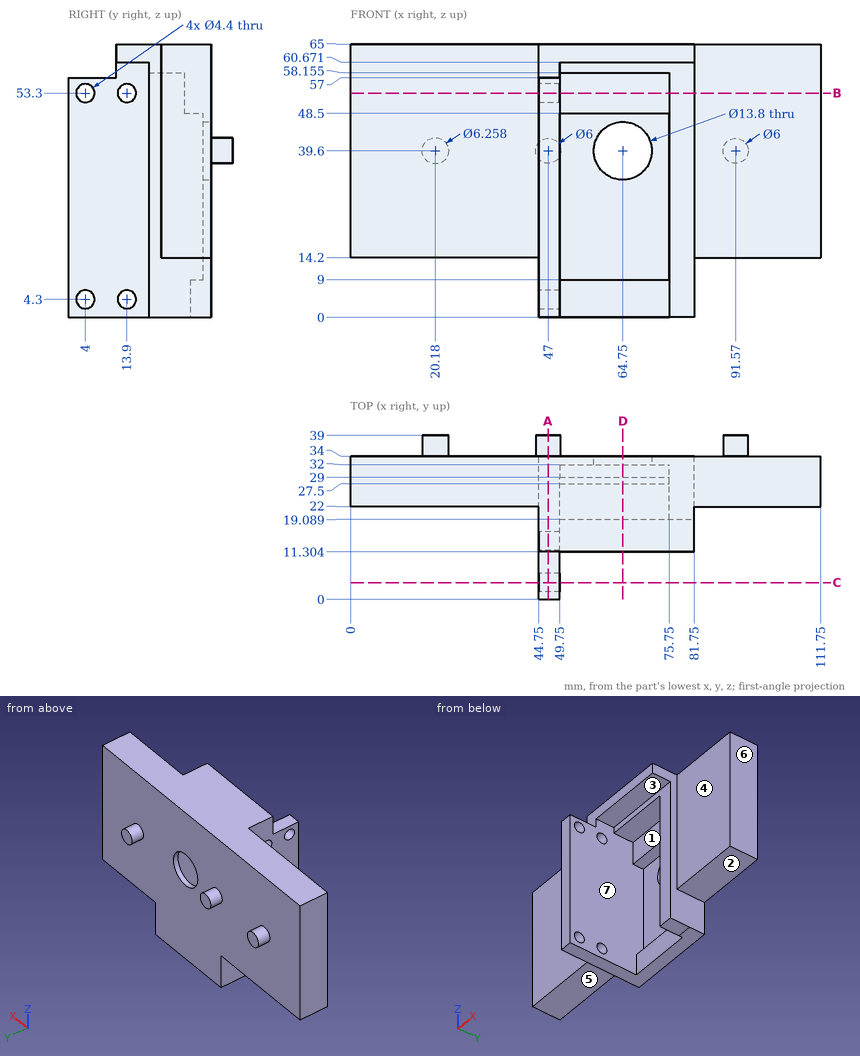
Geometry check sheet. Reference: drawing and pictorial views, mm from the part's lowest x, y, z. A direction names the side the tool comes from. Round coordinates to 2 decimals unless told otherwise and drop trailing zeros. Write each loop counter-clockwise with the first axis right and the second up, starting at its lowest first coordinate (ties: lowest second). Pieces come first, ordered by that corner, then holes. Notation, with made-up numbers: (37.25, 61) -> (66.25, 61) arc R21 cw to (66.25, 88) -> close; hole circle Ø10 at (74.5, -2). An arc over 180 degrees is marked (long way). Answer as CSV lines item,"result". Start each with the question number.
1) Tool access check on the marked faces 1, 2, 3 and 4. Record the directions out of +Z, -Z, +X, -X, +Y, -Y that give a thin tool (end or side, any length) a straight path to the whole face; none if there is none.
2) Material ranges on line 1 (Y direction, x = 46, z = 53); line 2 (X direction, y = 19.5, z = 10); line 3 (X direction, y = 26.5, z = 24.5), recorded low to high. Write a range as from..to.
3) Release check for a two-part mould opening along X. For the marked faces 5, 6 and 7 record: pulls with the +X half, pulls with the -X half, needs draft (parallel to the pull), parting line crosses it, or undercut.
4) Section check B-B on z = 53.3. Enter the section's corners in (x, y).
5) Section check A-A on x = 47. Enter the section's corners in (y, z).
6) Go/stop test with flat-tipped pins: P1, Ø4.5, axis at x = 57, z = 4, coming from the -Y side; P2, Ø4, axis at y = 13.9, z = 4.3, coming from the -X side; P3, Ø3.5, axis at x = 102.5, y = 30, coming from the -Z side; P4, Ø16, axis at x = 66, z = 32.5, coming from the -Y side. Record where each tip stops, or that it passes through.
7) Section check C-C on y = 4. Enter the section's corners in (x, z), and give its area (3 significant figures).
8) Section check D-D on x = 64.75. Enter the section's corners in (y, z) (1 decimal), and give its area (3 significant figures).
Found:
1,face 1,"-Z, -Y"
1,face 2,"-Z, +X, +Y, -Y"
1,face 3,"-Z, +X, -Y"
1,face 4,"+Z, -Z, +X, -Y"
2,line 1,"y = 0..1.82, 6.18..11.72, 16.08..34"
2,line 2,"x = 44.75..49.75, 75.75..81.75"
2,line 3,"x = 0..49.75, 75.75..111.75"
3,face 5,"needs draft"
3,face 6,"pulls with the +X half"
3,face 7,"undercut"
4,outline,"(0, 22) -> (44.75, 22) -> (44.75, 16.1) -> (49.75, 16.1) -> (49.75, 27.5) -> (75.75, 27.5) -> (75.75, 19.09) -> (81.75, 19.09) -> (81.75, 22) -> (111.75, 22) -> (111.75, 34) -> (0, 34) -> close; (44.75, 0) -> (49.75, 0) -> (49.75, 1.8) -> (44.75, 1.8) -> close; (44.75, 6.2) -> (49.75, 6.2) -> (49.75, 11.7) -> (44.75, 11.7) -> close"
5,outline,"(0, 0) -> (34, 0) -> (34, 36.6) -> (39, 36.6) -> (39, 42.6) -> (34, 42.6) -> (34, 65) -> (11.3, 65) -> (11.3, 57) -> (0, 57) -> close; hole circle Ø4.4 at (4, 4.3); hole circle Ø4.4 at (4, 53.3); hole circle Ø4.4 at (13.9, 4.3); hole circle Ø4.4 at (13.9, 53.3)"
6,P1,"stops at y = 29"
6,P2,"passes through"
6,P3,"stops at z = 14.2"
6,P4,"stops at y = 32"
7,outline,"(44.75, 0) -> (49.75, 0) -> (49.75, 2.1) -> (44.75, 2.1) -> close; (44.75, 6.5) -> (49.75, 6.5) -> (49.75, 51.1) -> (44.75, 51.1) -> close; (44.75, 55.5) -> (49.75, 55.5) -> (49.75, 57) -> (44.75, 57) -> close"
7,area,"241 mm^2"
8,outline,"(11.3, 60.7) -> (19.1, 60.7) -> (19.1, 58.2) -> (27.5, 58.2) -> (27.5, 48.5) -> (32, 48.5) -> (32, 46.5) -> (34, 46.5) -> (34, 65) -> (11.3, 65) -> close; (29, 0) -> (34, 0) -> (34, 32.7) -> (32, 32.7) -> (32, 9) -> (29, 9) -> close"
8,area,"295 mm^2"
